Verification items for the finished model (mm, model axes). A direction names the side the tool comes from. Round coordinates to 2 decimals unless told otherwise and drop trailing zeros. Order: outer loops, then holes, each group sorted by start corner. A loop starts at its lowest first (then second) coordinate and runs counter-clockwise, first axis right, second up. Notation, with made-up numbers: M 75.5,58.5 L 126.5,58.5 A4 ccw 126.5,62.5 Z; hole C 29.5,86 d1. An arc over 180 degrees is marked long. Use CSV: the item, a comma, the result in double quotes. Start each with the question number.
Q1. Set-up check for faces 1 (the face through (17, -11, -17)), 2 (the face through (0, -1, -6.75)), 3 (the face through (36, -3, -5)): record each of +Z, -Z, +X, -X, +Y, -Y from which the full face is reachable in a straight line by a thin tool's end or side.
Q2. Scan lines: line 1 (X direction, y = -10.75, z = 19); line 2 (X direction, y = -1, z = 23); line 3 (Z direction, x = 27.5, y = -4.5). Record each from-to range of solid material in increasing order.
Q3. Sectioned sample at B-B (z = 19). Enter the section's corners in (x, y).
Q4. Sectioned sample at A-A (x = -19). State how many separate pieces and enclosed holes the cut face has, and give its area (3 significant figures).
Q5. Sectioned sample at D-D (z = -34). Enter the section's corners in (x, y), and give its area (3 significant figures).
Q6. Mould release check, pull along X, two halves, no side actions. Record for faces 4 (the face through (-14, -8, 14)), 5 (the face through (-36, -2, 5)), 6 (the face through (-18.83, -10.67, 5.54)): +X half, -X half, draft (parallel to the pull), parting line (faces both ways), or undercut.
Q7. Gauge pin test, flat ends, axial feed: pin 1 Ø7.5 at (x, z) = (-19, -19) entering from +Y; pin 2 Ø4 at (x, z) = (22.5, 25.5) entering from +Y; pin 3 Ø1.5 at (y, z) = (-12, 16) entering from -X; pin 4 Ø2 at (x, z) = (26, -1.5) entering from +Y. Record the tip position at first contact, or that the pin passes through.
```python
from build123d import *

# Parameters (mm, degrees)
SKETCH1_W               = 80
SKETCH1_H               = 80
BOSS_EXTRUDE1_DEPTH     = 16
CUT_EXTRUDE1_DEPTH      = 59.787753827
CUT_EXTRUDE1_DEPTH_BACK = 59.787753827
SKETCH2_R               = 1.75
SKETCH3_W               = 24.5
SKETCH3_H               = 15.5
CUT_EXTRUDE2_DEPTH      = 13
FILLET1_R               = 7.75
SKETCH4_W               = 15.5
SKETCH4_H               = 24.5
CUT_EXTRUDE3_DEPTH      = 3
BOSS_EXTRUDE2_DEPTH     = 23.5
CUT_EXTRUDE4_DEPTH      = 59.787753827
CUT_EXTRUDE4_DEPTH_BACK = 59.787753827
CUT_EXTRUDE5_DEPTH      = 59.787753827
CUT_EXTRUDE5_DEPTH_BACK = 59.787753827
SKETCH7_R               = 10
CUT_EXTRUDE6_DEPTH      = 59.787753827
CUT_EXTRUDE6_DEPTH_BACK = 59.787753827
CHAMFER1_SIZE           = 4
CHAMFER2_SIZE           = 30
BOSS_EXTRUDE4_START     = -3
SKETCH11_R              = 10
SKETCH11_R_2            = 4.25
BOSS_EXTRUDE4_DEPTH     = 3
SKETCH12_R              = 4
CUT_EXTRUDE7_DEPTH      = 5
CUT_EXTRUDE8_START      = -10
SKETCH13_R              = 3
SKETCH13_R_2            = 1.75
CUT_EXTRUDE8_DEPTH      = 10


with BuildPart() as part:
    # Sketch1 → Boss-Extrude1 (new body)
    with BuildSketch(Plane(origin=(0, 0, 0), x_dir=(1, 0, 0), z_dir=(0, 1, 0))):
        Rectangle(SKETCH1_W, SKETCH1_H)
    extrude(amount=-BOSS_EXTRUDE1_DEPTH)

    # Sketch2 → Cut-Extrude1 (cut, two sides: drawn at the far end of the back side and taken through both)
    with BuildSketch(Plane(origin=(0, 0, 0), x_dir=(1, 0, 0), z_dir=(0, 1, 0)).offset(-CUT_EXTRUDE1_DEPTH_BACK)):
        with Locations(Location((-11.5, -11.5, 0), (0, 0, 270))):
            Circle(SKETCH2_R)
        with Locations(Location((11.5, 11.5, 0), (0, 0, 270))):
            Circle(SKETCH2_R)
        with Locations(Location((22, 22, 0), (0, 0, 270))):
            Circle(SKETCH2_R)
        with Locations(Location((19, -34.5, 0), (0, 0, 270))):
            Circle(SKETCH2_R)
        with Locations(Location((34.5, -19, 0), (0, 0, 270))):
            Circle(SKETCH2_R)
        with Locations(Location((-34.5, 19, 0), (0, 0, 270))):
            Circle(SKETCH2_R)
        with Locations(Location((-19, 34.5, 0), (0, 0, 270))):
            Circle(SKETCH2_R)
    extrude(amount=CUT_EXTRUDE1_DEPTH + CUT_EXTRUDE1_DEPTH_BACK, mode=Mode.SUBTRACT)

    # Sketch3 → Cut-Extrude2 (cut)
    with BuildSketch(Plane(origin=(0, 0, 0), x_dir=(1, 0, 0), z_dir=(0, 1, 0))):
        with Locations((19, 0)):
            Rectangle(SKETCH3_W, SKETCH3_H)
        with Locations((-19, 0)):
            Rectangle(SKETCH3_W, SKETCH3_H)
    extrude(amount=-CUT_EXTRUDE2_DEPTH, mode=Mode.SUBTRACT)

    # Fillet1
    fillet1_edges = [part.edges().sort_by_distance(p)[0] for p in [
        (19, -13, 7.75),
        (19, -13, -7.75),
        (-19, -13, 7.75),
        (-19, -13, -7.75),
    ]]
    fillet(fillet1_edges, radius=FILLET1_R - 0.0001)  # a hair under: the kernel refuses the full size

    # Sketch4 → Cut-Extrude3 (cut)
    with BuildSketch(Plane(origin=(0, 0, 0), x_dir=(1, 0, 0), z_dir=(0, 1, 0))):
        with Locations((0, -19)):
            Rectangle(SKETCH4_W, SKETCH4_H)
        with Locations((0, 19)):
            Rectangle(SKETCH4_W, SKETCH4_H)
    extrude(amount=-CUT_EXTRUDE3_DEPTH, mode=Mode.SUBTRACT)

    # Sketch5 → Boss-Extrude2 (add)
    with BuildSketch(Plane(origin=(0, 0, 31.25), x_dir=(-1, 0, 0), z_dir=(0, 0, -1))):
        with BuildLine():
            ThreePointArc((-8e-09, -3), (-3.409545428, -2.209705452), (-6.123724357, 0))
            Line((-6.123724357, 0), (-7.75, 0))
            Line((-7.75, 0), (-7.75, -3))
            Line((-7.75, -3), (-8e-09, -3))
        make_face()
        with BuildLine():
            Line((7.75, -3), (7.75, 0))
            Line((7.75, 0), (6.123724357, 0))
            ThreePointArc((6.123724357, 0), (3.409545421, -2.209705455), (-8e-09, -3))
            Line((-8e-09, -3), (7.75, -3))
        make_face()
    boss_extrude2 = extrude(amount=BOSS_EXTRUDE2_DEPTH)

    # Mirror1: Boss-Extrude2 across plane
    add(boss_extrude2.mirror(Plane.XY))

    # Sketch6 → Cut-Extrude4 (cut, two sides: drawn at the far end of the back side and taken through both)
    with BuildSketch(Plane(origin=(0, 0, 0), x_dir=(0, 0, -1), z_dir=(1, 0, 0)).offset(-CUT_EXTRUDE4_DEPTH_BACK)):
        with BuildLine():
            ThreePointArc((-5, -5), (0, -10), (5, -5))
            Line((5, -5), (-5, -5))
        make_face()
        with BuildLine():
            Line((-5, -5), (5, -5))
            ThreePointArc((5, -5), (3.535533906, -1.464466094), (0, 0))
            ThreePointArc((0, 0), (-3.535533906, -1.464466094), (-5, -5))
        make_face()
        with BuildLine():
            Line((-5, 0), (-5, -5))
            ThreePointArc((-5, -5), (-3.535533906, -1.464466094), (0, 0))
            Line((0, 0), (-5, 0))
        make_face()
        with BuildLine():
            ThreePointArc((0, 0), (3.535533906, -1.464466094), (5, -5))
            Line((5, -5), (5, 0))
            Line((5, 0), (0, 0))
        make_face()
    extrude(amount=CUT_EXTRUDE4_DEPTH + CUT_EXTRUDE4_DEPTH_BACK, mode=Mode.SUBTRACT)

    # Sketch7 → Cut-Extrude5 (cut, two sides: drawn at the far end of the back side and taken through both)
    with BuildSketch(Plane(origin=(0, 0, 0), x_dir=(1, 0, 0), z_dir=(0, 1, 0)).offset(-CUT_EXTRUDE5_DEPTH_BACK)):
        with Locations(Location((19, -19, 0), (0, 0, 270))):
            Circle(SKETCH7_R)
        with Locations(Location((-19, 19, 0), (0, 0, 270))):
            Circle(SKETCH7_R)
    extrude(amount=CUT_EXTRUDE5_DEPTH + CUT_EXTRUDE5_DEPTH_BACK, mode=Mode.SUBTRACT)

    # Sketch9 → Cut-Extrude6 (cut, two sides: drawn at the far end of the back side and taken through both)
    with BuildSketch(Plane(origin=(0, 0, 0), x_dir=(1, 0, 0), z_dir=(0, 1, 0)).offset(-CUT_EXTRUDE6_DEPTH_BACK)):
        Polygon((-10, -18), (-18, -10), (-18, -18), align=None)
        Polygon((-10, -40), (-10, -18), (-18, -18), (-18, -10), (-40, -10), (-40, -40), align=None)
    extrude(amount=CUT_EXTRUDE6_DEPTH + CUT_EXTRUDE6_DEPTH_BACK, mode=Mode.SUBTRACT)

    # Chamfer1
    chamfer1_edges = [part.edges().sort_by_distance(p)[0] for p in [
        (-10, -8, 40),
        (-40, -8, 10),
        (40, -8, 40),
        (-40, -8, -40),
    ]]
    chamfer(chamfer1_edges, length=CHAMFER1_SIZE)

    # Chamfer2
    chamfer2_edges = [part.edges().sort_by_distance(p)[0] for p in [
        (40, -8, -40),
    ]]
    chamfer(chamfer2_edges, length=CHAMFER2_SIZE)

    # Sketch11 → Boss-Extrude4 (add)
    # profile 1 of 2: a face of its own
    with BuildSketch(Plane.XZ.offset(16).offset(BOSS_EXTRUDE4_START)):
        with Locations(Location((-19, -19, 0), (0, 0, 270))):
            Circle(SKETCH11_R)
        with Locations(Location((-19, -19, 0), (0, 0, 270))):
            Circle(SKETCH11_R_2, mode=Mode.SUBTRACT)
    # profile 2 of 2: a face of its own
    with BuildSketch(Plane.XZ.offset(16).offset(BOSS_EXTRUDE4_START)):
        with Locations(Location((19, 19, 0), (0, 0, 270))):
            Circle(SKETCH11_R)
        with Locations(Location((19, 19, 0), (0, 0, 270))):
            Circle(SKETCH11_R_2, mode=Mode.SUBTRACT)
    extrude(amount=BOSS_EXTRUDE4_DEPTH)

    # Sketch12 → Cut-Extrude7 (cut)
    with BuildSketch(Plane.XZ.offset(16)):
        with Locations(Location((0, 0, 0), (0, 0, 270))):
            Circle(SKETCH12_R)
        with Locations(Location((16.75, -16.75, 0), (0, 0, 270))):
            Circle(SKETCH12_R)
    extrude(amount=-CUT_EXTRUDE7_DEPTH, mode=Mode.SUBTRACT)

    # Sketch13 → Cut-Extrude8 (cut)
    # profile 1 of 7: a face of its own
    with BuildSketch(Plane.XZ.offset(16).offset(CUT_EXTRUDE8_START)):
        with Locations(Location((19, 34.5, 0), (0, 0, 270))):
            Circle(SKETCH13_R)
        with Locations(Location((19, 34.5, 0), (0, 0, 270))):
            Circle(SKETCH13_R_2, mode=Mode.SUBTRACT)
    # profile 2 of 7: a face of its own
    with BuildSketch(Plane.XZ.offset(16).offset(CUT_EXTRUDE8_START)):
        with Locations(Location((34.5, 19, 0), (0, 0, 270))):
            Circle(SKETCH13_R)
        with Locations(Location((34.5, 19, 0), (0, 0, 270))):
            Circle(SKETCH13_R_2, mode=Mode.SUBTRACT)
    # profile 3 of 7: a face of its own
    with BuildSketch(Plane.XZ.offset(16).offset(CUT_EXTRUDE8_START)):
        with Locations(Location((-11.5, 11.5, 0), (0, 0, 270))):
            Circle(SKETCH13_R)
        with Locations(Location((-11.5, 11.5, 0), (0, 0, 270))):
            Circle(SKETCH13_R_2, mode=Mode.SUBTRACT)
    # profile 4 of 7: a face of its own
    with BuildSketch(Plane.XZ.offset(16).offset(CUT_EXTRUDE8_START)):
        with Locations(Location((-34.5, -19, 0), (0, 0, 270))):
            Circle(SKETCH13_R)
        with Locations(Location((-34.5, -19, 0), (0, 0, 270))):
            Circle(SKETCH13_R_2, mode=Mode.SUBTRACT)
    # profile 5 of 7: a face of its own
    with BuildSketch(Plane.XZ.offset(16).offset(CUT_EXTRUDE8_START)):
        with Locations(Location((-19, -34.5, 0), (0, 0, 270))):
            Circle(SKETCH13_R)
        with Locations(Location((-19, -34.5, 0), (0, 0, 270))):
            Circle(SKETCH13_R_2, mode=Mode.SUBTRACT)
    # profile 6 of 7: a face of its own
    with BuildSketch(Plane.XZ.offset(16).offset(CUT_EXTRUDE8_START)):
        with Locations(Location((11.5, -11.5, 0), (0, 0, 270))):
            Circle(SKETCH13_R)
        with Locations(Location((11.5, -11.5, 0), (0, 0, 270))):
            Circle(SKETCH13_R_2, mode=Mode.SUBTRACT)
    # profile 7 of 7: a face of its own
    with BuildSketch(Plane.XZ.offset(16).offset(CUT_EXTRUDE8_START)):
        with Locations(Location((22, -22, 0), (0, 0, 270))):
            Circle(SKETCH13_R)
        with Locations(Location((22, -22, 0), (0, 0, 270))):
            Circle(SKETCH13_R_2, mode=Mode.SUBTRACT)
    extrude(amount=CUT_EXTRUDE8_DEPTH, mode=Mode.SUBTRACT)


solid = part.part
```
Verdict:
1,face 1,"-Y"
1,face 2,"+Y"
1,face 3,"+X, -X, +Y"
2,line 1,"x = -10 to 9, 29 to 31.5, 37.5 to 40"
2,line 2,"x = -10 to -5.2, 5.2 to 9.83, 28.17 to 40"
2,line 3,"z = -22.5 to -7.75, 7.75 to 13.73, 24.27 to 40"
3,outline,"M -10,-16 L 14.75,-16 L 14.75,-13 L 9,-13 L 9,0 L 6.12,0 A7.75 cw -6.12,0 L -10,0 Z; M 23.25,-16 L 31.5,-16 L 31.5,-6 L 32.75,-6 L 32.75,0 L 29,0 L 29,-13 L 23.25,-13 Z; M 36.25,-6 L 37.5,-6 L 37.5,-16 L 40,-16 L 40,0 L 36.25,0 Z"
4,separate pieces,"3"
4,enclosed holes,"0"
4,area,"258 mm²"
5,outline,"M -40,-16 L -21.96,-16 L -21.96,-6 L -20.68,-6 L -20.68,0 L -40,0 Z; M -17.32,-6 L -16.04,-6 L -16.04,-16 L 16,-16 L 16,0 L -17.32,0 Z"
5,area,"817 mm²"
6,face 4,"-X half"
6,face 5,"draft"
6,face 6,"undercut"
7,pin 1,"passes through"
7,pin 2,"stops at y = -13"
7,pin 3,"stops at x = -12.75"
7,pin 4,"stops at y = -12.59"
